Can you work these out from the model? Positions are in its coordinate system, mm. A direction names the side the tool comes from. Give positions to 0.01 mm unless a question says otherwise; leave off trailing zeros. Loops run counter-clockwise (first coordinate to the right, second up) from the corner with the lowest first, then second, coordinate; pieces in that order, holes last.
from build123d import *

# Parameters (mm, degrees)
F0_W      = 20
F0_H      = 105
F1_DEPTH  = 1000
F2_W      = 1060
F2_H      = 105
F3_DEPTH  = 20
F4_W      = 1175
F4_H      = 155
F5_DEPTH  = 20
F7_W      = 508
F7_H      = 35
F8_DEPTH  = 1040
F9_DEPTH  = 475
F11_DEPTH = 10
F13_DEPTH = 1020
F15_DEPTH = 10
F16_SIZE2 = 9.99999
F16_SIZE  = 4.99999


# Not quite as in the source:
# - a fillet or chamfer is up to 0.001 mm smaller than in the source, because OpenCascade refuses the exact size


with BuildPart() as f1:
    # F0 (on Top) → F1 (new body)
    with BuildSketch(Plane.XY):
        with Locations((-520, -52.5)):
            Rectangle(F0_W, F0_H)
    extrude(amount=F1_DEPTH)



with BuildPart() as f1b:
    # F0 (on Top) → F1, piece 2 (new body)
    with BuildSketch(Plane.XY):
        with Locations((520, -52.5)):
            Rectangle(F0_W, F0_H)
    extrude(amount=F1_DEPTH)


with BuildPart() as f1c:
    # F0 (on Top) → F1, piece 3 (new body)
    with BuildSketch(Plane.XY):
        Polygon((35, 0), (0, 0), (-35, 0), (-35, -70), (-25, -80), (25, -80), (35, -70), align=None)
    extrude(amount=F1_DEPTH)


with BuildPart() as f1_1:
    add(f1.part)

    add(f1b.part)  # F3 merges F1b

    add(f1c.part)  # F3 merges F1c
    # F2 (on face) → F3 (join)
    with BuildSketch(Plane.XY.offset(1000)):
        with Locations((0, -52.5)):
            Rectangle(F2_W, F2_H)
    extrude(amount=F3_DEPTH)

    # F4 (on face) → F5 (join)
    with BuildSketch(Plane(origin=(0, 0, 0), x_dir=(1, 0, 0), z_dir=(0, 0, -1))):
        with Locations((0, 77.5)):
            Rectangle(F4_W, F4_H)
    extrude(amount=F5_DEPTH)

    # F7 (on face) → F8 (cut, through all)
    with BuildSketch(Plane.XY.offset(1020)):
        with Locations((-276, -17.5)):
            Rectangle(F7_W, F7_H)
    extrude(amount=-F8_DEPTH, mode=Mode.SUBTRACT)

    # F6 (on face) → F9 (join, through all)
    with BuildSketch(Plane(origin=(510, 0, 0), x_dir=(0, -1, 0), z_dir=(-1, 0, 0))):
        Polygon((0, 55), (0, 0), (30, 0), (30, 45), (15, 55), align=None)
    extrude(amount=F9_DEPTH)

    # F10 (on face) → F11 (join)
    with BuildSketch(Plane.XZ.offset(105)):
        Polygon((515, 1005), (515, 0), (535, 0), (535, 1025), (-535, 1025), (-535, 0), (-515, 0), (-515, 1005), align=None)
    extrude(amount=F11_DEPTH)

    # F12 (on Top) → F13 (join, through all)
    with BuildSketch(Plane.XY):
        Polygon((-20, 0), (0, 0), (20, 0), (20, 15), (-20, 15), align=None)
    extrude(amount=F13_DEPTH)

    # F14 (on face) → F15 (join)
    with BuildSketch(Plane.XZ.offset(115)):
        Polygon((520, 1010), (520, 0), (580, 0), (580, 1070), (-580, 1070), (-580, 0), (-520, 0), (-520, 1010), align=None)
    extrude(amount=F15_DEPTH)

    # F16 (size 5 and 10 in the source; OpenCascade refuses exactly that, so slightly less here)
    f16_edges = [f1_1.edges().sort_by_distance(p)[0] for p in [
        (-520, -125, 505),
        (0, -125, 1010),
        (520, -125, 505),
    ]]
    f16_side = f1_1.faces().sort_by_distance((535.781318, -125, 505))[0]
    chamfer(f16_edges, length=F16_SIZE, length2=F16_SIZE2, reference=f16_side)


solid = f1_1.part
(1) Which directions (+Z, -Z, +X, -X, +Y, -Y) give clear straight access to the entire face, cutting with the end or side of a thin tool? Please do faces 1 (the flat face through (276, -30, 22)), 2 (the flat face through (-35, -52, 493)), 3 (the flat face through (-7, -57, 1020)), 4 (the flat face through (530, -53, 503)).
Returned:
face 1: -Y
face 2: +Y, -Y
face 3: +Z, +X, -X, +Y
face 4: +Z, +X, +Y
(2) Thinking about a two-plate mould opening in Z: for faces 5 (the flat face through (-3, -115, 1053)), 6 (the flat face through (-8, -79, -20)), 7 (the flat face through (35, -35, 493)), which applies, pulls with the +Z half, pulls with the -Z half, needs draft (parallel to the pull), parting line crosses it, or undercut?
Returned:
face 5: needs draft
face 6: pulls with the -Z half
face 7: undercut
(3) Suppose I cut it at B-B on y = -54.5. List the corners of the cut face in (x, z) for me.
Returned:
outline: (-587.5, -20) - (587.5, -20) - (587.5, 0) - (530, 0) - (530, 1020) - (-530, 1020) - (-530, 0) - (-587.5, 0) - close; hole (-510, 0) - (-35, 0) - (-35, 1000) - (-510, 1000) - close; hole (35, 0) - (510, 0) - (510, 1000) - (35, 1000) - close
(4) Will these pins go through, and if not, where does the flat tip stop? P1, Ø7.5, axis at y = 7, z = 400, coming from the +X side; P2, Ø3, axis at y = -111, z = 373, coming from the +X side; P3, Ø5, axis at y = -71, z = 326.5, coming from the -X side.
Returned:
P1: stops at x = 20
P2: stops at x = 535
P3: stops at x = -530
(5) Suppose I cut it at C-C on z = 882.5. Give the number of separate pieces and of enclosed holes in the cut face, plus the area to 3 significant figures.
Returned:
separate pieces: 3
enclosed holes: 0
area: 10,700 mm2
(6) Please list where these lines run through material, in increasing order: probe 1 along X at (y, z) = (-70, 788.5); probe 2 along Z at (x, y) = (-179, -71.5); probe 3 along X at (y, z) = (-110, 107.5).
Returned:
probe 1: x = -530 to -510, -35 to 35, 510 to 530
probe 2: z = -20 to 0, 1000 to 1020
probe 3: x = -535 to -515, 515 to 535
